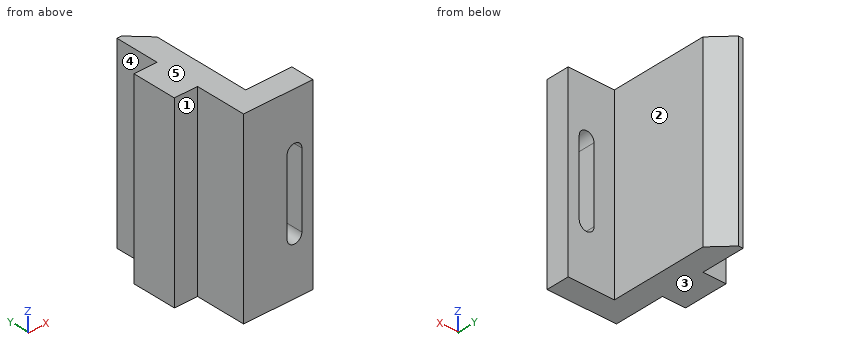
from build123d import *

# Parameters (mm, degrees)
BOSS_EXTRUDE1_DEPTH = 12.7
SKETCH2_W           = 3.175
SKETCH2_H           = 6.096
BOSS_EXTRUDE2_DEPTH = 12.7
CUT_EXTRUDE1_DEPTH  = 4.175
CHAMFER1_SIZE       = 2.54


with BuildPart() as part:
    # Sketch1 → Boss-Extrude1 (new body, symmetric)
    with BuildSketch(Plane.XY):
        Polygon((0, 0), (9.525, 0), (9.525, 3.175), (3.175, 3.175), (3.175, 19.05), (0, 19.05), align=None)
    extrude(amount=BOSS_EXTRUDE1_DEPTH, both=True)

    # Sketch2 → Boss-Extrude2 (add, symmetric)
    with BuildSketch(Plane.XY):
        with Locations((-1.5875, 9.9822)):
            Rectangle(SKETCH2_W, SKETCH2_H)
    extrude(amount=BOSS_EXTRUDE2_DEPTH, both=True)

    # Sketch3 → Cut-Extrude1 (cut, through all)
    with BuildSketch(Plane(origin=(0, 3.175, 0), x_dir=(1, 0, 0), z_dir=(0, 1, 0))):
        with BuildLine():
            Line((8.001, 5.08), (8.001, -5.08))
            ThreePointArc((8.001, -5.08), (6.985, -6.096), (5.969, -5.08))
            Line((5.969, -5.08), (5.969, 5.08))
            ThreePointArc((5.969, 5.08), (6.985, 6.096), (8.001, 5.08))
        make_face()
    extrude(amount=-CUT_EXTRUDE1_DEPTH, mode=Mode.SUBTRACT)

    # Chamfer1
    chamfer1_edges = [part.edges().sort_by_distance(p)[0] for p in [
        (3.175, 19.05, 0),
    ]]
    chamfer(chamfer1_edges, length=CHAMFER1_SIZE)


solid = part.part
Build history of the part. All positions in model axes, mm. Face numbers are marked on the shaded views. A direction names the side the tool comes from. Coordinates: 2 decimals unless noted, no trailing zeros. Write each loop counter-clockwise with the first axis right and the second up, starting at its lowest first coordinate (ties: lowest second). Pieces come first, ordered by that corner, then holes. Notation, with made-up numbers: (50, 76) -> (72, 76) arc R21 cw to (72, 108) -> close; hole circle Ø6 at (-25, 25.25). An arc over 180 degrees is marked (long way). Use CSV: the item, a comma, the result in double quotes. Start each with the question number.
Q1. Cut at C-C, the plane x = 6.5. List the corners of the cut face in (y, z) (3 decimals).
Q2. Cut at B-B, the plane y = 2.5. List the corners of the cut face in (x, z) (3 decimals), then the cut area to 3 significant figures.
Q3. Drill centre lines: probe 1 along X at (y, z) = (2.75, 3.5) (3 decimals); probe 2 along Y at (x, z) = (5.75, 4.75) (3 decimals). Where is each one in solid material? Low to high.
Q4. Cut at D-D, the plane z = -9.5. List the corners of the cut face in (x, y) (3 decimals), then the cut area to 3 significant figures.
Q5. Flat gauge pins, fed straight in: pin 1 Ø10 at (y, z) = (17, 3.5) entering from +X (3 decimals); pin 2 Ø2.5 at (x, z) = (-1.5, 4.5) entering from +Y; pin 3 Ø1.9 at (x, z) = (7.5, -2) entering from +Y (3 decimals). Where does each tip first touch, or does it go through?
Q6. 3-axis set-ups, long thin cutter, end or side, ignore diameter. For the marked faces 1, 2, 3, 4 and 5: which of +Z, -Z, +X, -X, +Y, -Y reach the whole face in a straight line?
Q7. Cut at A-A, the plane z = -4.25. List the corners of the cut face in (x, y) (3 decimals), then the cut area to 3 significant figures.
Checked values:
1,outline,"(0, -12.7) -> (3.175, -12.7) -> (3.175, -5.973) -> (0, -5.973) -> close; (0, 5.973) -> (3.175, 5.973) -> (3.175, 12.7) -> (0, 12.7) -> close"
2,outline,"(0, -12.7) -> (9.525, -12.7) -> (9.525, 12.7) -> (0, 12.7) -> close; hole (5.969, -5.08) arc R1.016 ccw to (8.001, -5.08) -> (8.001, 5.08) arc R1.016 ccw to (5.969, 5.08) -> close"
2,area,"218 mm²"
3,probe 1,"x = 0 to 5.969, 8.001 to 9.525"
3,probe 2,"y = 0 to 3.175"
4,outline,"(-3.175, 6.934) -> (0, 6.934) -> (0, 0) -> (9.525, 0) -> (9.525, 3.175) -> (3.175, 3.175) -> (3.175, 16.51) -> (0.635, 19.05) -> (0, 19.05) -> (0, 13.03) -> (-3.175, 13.03) -> close"
4,area,"96.8 mm²"
5,pin 1,"stops at x = 3.175"
5,pin 2,"stops at y = 13.03"
5,pin 3,"stops at y = 3.175"
6,face 1,"+Z, -Z, -X, -Y"
6,face 2,"+Z, -Z, +X, +Y"
6,face 3,"-Z, +X, -X, +Y, -Y"
6,face 4,"+Z, -Z, -X, +Y"
6,face 5,"+Z, +X, -X, +Y, -Y"
7,outline,"(-3.175, 6.934) -> (0, 6.934) -> (0, 0) -> (5.969, 0) -> (5.969, 3.175) -> (3.175, 3.175) -> (3.175, 16.51) -> (0.635, 19.05) -> (0, 19.05) -> (0, 13.03) -> (-3.175, 13.03) -> close; (8.001, 0) -> (9.525, 0) -> (9.525, 3.175) -> (8.001, 3.175) -> close"
7,area,"90.3 mm²"
